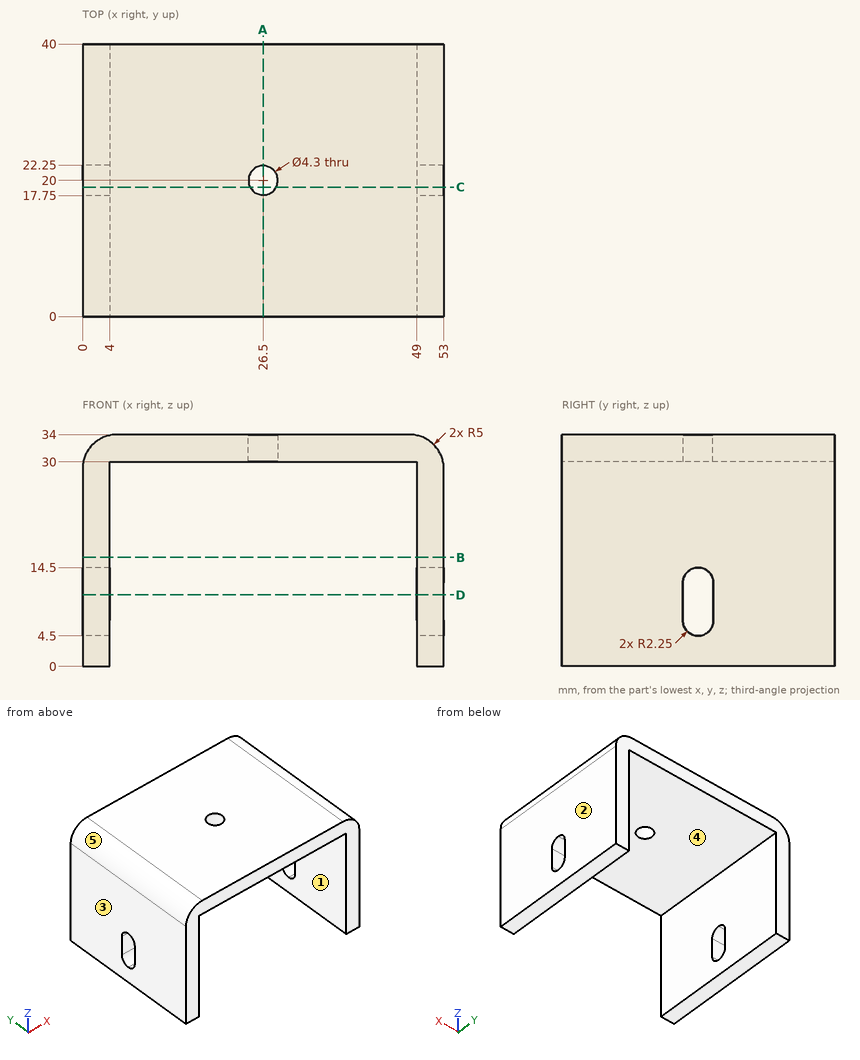
Check sheet for the drawn part. Datum: minimum x, y, z corner. Units: mm. A direction names the side the tool comes from. Give positions to 0.01 mm unless a question says otherwise; leave off trailing zeros. Order: outer loops, then holes, each group sorted by start corner. A loop starts at its lowest first (then second) coordinate and runs counter-clockwise, first axis right, second up.
1. Sectioned sample at B-B (z = 16). Record the boundary of the cut face in (x, y).
Completed:
outline: (0, 0) - (4, 0) - (4, 40) - (0, 40) - close; (49, 0) - (53, 0) - (53, 40) - (49, 40) - close
2. Depth check by flat-ended pin: pin 1 (1 mm diameter, centred on y = 10.5, z = 29.5, fed in from +X); pin 2 (12 mm diameter, centred on x = 31, y = 27.5, fed in from -Z). Enter the tip coordinate at first touch or a pass-through.
Completed:
pin 1: stops at x = 53
pin 2: stops at z = 30
3. Sectioned sample at A-A (x = 26.5). Record the boundary of the cut face in (y, z).
Completed:
outline: (0, 30) - (17.85, 30) - (17.85, 34) - (0, 34) - close; (22.15, 30) - (40, 30) - (40, 34) - (22.15, 34) - close
4. Access from +Z, -Z, +X, -X, +Y, -Y to the whole of each face (thin tool, end or side, straight path). Record for the marked faces 4 and 5.
Completed:
face 4: -Z, +Y, -Y
face 5: +Z, -X, +Y, -Y
5. Scan lines: line 1 (X direction, y = 8.5, z = 27.5); line 2 (Y direction, x = 26.5, z = 31.85); line 3 (Z direction, x = 45.5, y = 25). Record each from-to range of solid material in increasing order.
Completed:
line 1: x = 0 to 4, 49 to 53
line 2: y = 0 to 17.85, 22.15 to 40
line 3: z = 30 to 34
6. Draft check along X on the marked faces 1, 2 and 3. Enter one of: pulls with the +X half, pulls with the -X half, needs draft (parallel to the pull), parting line crosses it, or undercut.
Completed:
face 1: undercut
face 2: pulls with the +X half
face 3: pulls with the -X half
7. Sectioned sample at D-D (z = 10.5). Record the boundary of the cut face in (x, y), then the cut area to 3 significant figures.
Completed:
outline: (0, 0) - (4, 0) - (4, 17.75) - (0, 17.75) - close; (0, 22.25) - (4, 22.25) - (4, 40) - (0, 40) - close; (49, 0) - (53, 0) - (53, 17.75) - (49, 17.75) - close; (49, 22.25) - (53, 22.25) - (53, 40) - (49, 40) - close
area: 284 mm2
8. Sectioned sample at C-C (y = 19). Record the boundary of the cut face in (x, z), then the cut area to 3 significant figures.
Completed:
outline: (0, 0) - (4, 0) - (4, 4.73) - (0, 4.73) - close; (0, 14.27) - (4, 14.27) - (4, 30) - (24.6, 30) - (24.6, 34) - (5, 34) arc R5 ccw to (0, 29) - close; (28.4, 30) - (49, 30) - (49, 14.27) - (53, 14.27) - (53, 29) arc R5 ccw to (48, 34) - (28.4, 34) - close; (49, 0) - (53, 0) - (53, 4.73) - (49, 4.73) - close
area: 350 mm2
